The model under review builds one solid part; all positions refer to its coordinate system, in mm. Round coordinates to 2 decimals unless told otherwise and drop trailing zeros. Loops run counter-clockwise (first coordinate to the right, second up) from the corner with the lowest first, then second, coordinate; pieces in that order, holes last. Notation, with made-up numbers: (36, 14.25) -> (84, 14.25) arc R19 cw to (84, 24.25) -> close; hole circle Ø8 at (65, 22.5). An arc over 180 degrees is marked (long way). Use a Markdown table: item, result. Add a question column.
1) Wall thickness on probe 1 along Z at (x, y) = (-1, 1.25); probe 2 along Y at (x, z) = (7, 2.35); probe 3 along Y at (x, z) = (12, 0.95): over which ranges is each line inside the solid? List them lowest first.
2) Insertion check: pin 1 (2 mm diameter, centred on x = -9.5, y = -7.5, fed in from +Z); pin 2 (1 mm diameter, centred on y = 9.5, z = 1.5, fed in from +X); pin 3 (0.7 mm diameter, centred on x = -24, z = 1, fed in from -Y). Each pin has a flat end and moves straight along its axis. Give the tip position at first contact, or say it passes through.
3) Consider section B-B on x = -2. Give the boundary of the cut face in (y, z), plus the area to 3 significant figures.
4) Consider section A-A on x = -11. Give the boundary of the cut face in (y, z).
5) Mouldability with a two-part tool opening along X and no side actions: class faces 1 (the cylindrical face through (-21.37, -2.9, 0.8)), 2 (the flat face through (1, 0, 0)) as released by +X, released by -X, zero draft, split by the parting line, or undercut.
from build123d import *

# Parameters (mm, degrees)
SKETCH_W      = 7
SKETCH_H      = 7
PAD_DEPTH     = 2
FILLET_R      = 4
FILLET001_R   = 8
FILLET002_R   = 2
FILLET003_R   = 3
SKETCH001_W   = 33
SKETCH001_H   = 2
SKETCH001_W_2 = 4
PAD001_DEPTH  = 1
FILLET004_R   = 4
CHAMFER_SIZE  = 0.9
FILLET005_R   = 0.9
FILLET006_R   = 0.9
FILLET007_R   = 0.9
FILLET008_R   = 0.5
FILLET009_R   = 0.5
FILLET010_R   = 0.5


with BuildPart() as part:
    # Sketch → Pad (new body)
    with BuildSketch(Plane.XY):
        Polygon((-11.80015, 8), (32.19985, 8), (32.19985, -8), (-11.80015, -8), (-11.80015, -14), (-30.80015, -14), (-30.80015, 14), (-11.80015, 14), align=None)
        with Locations((-24.30015, 0)):
            Rectangle(SKETCH_W, SKETCH_H, mode=Mode.SUBTRACT)
    extrude(amount=PAD_DEPTH)

    # Fillet
    fillet_edges = [part.edges().sort_by_distance(p)[0] for p in [
        (-11.80015, -14, 1),
        (-11.80015, 14, 1),
    ]]
    fillet(fillet_edges, radius=FILLET_R)

    # Fillet001
    fillet001_edges = [part.edges().sort_by_distance(p)[0] for p in [
        (-30.80015, -14, 1),
        (-30.80015, 14, 1),
    ]]
    fillet(fillet001_edges, radius=FILLET001_R)

    # Fillet002
    fillet002_edges = [part.edges().sort_by_distance(p)[0] for p in [
        (-20.80015, -3.5, 1),
        (-20.80015, 3.5, 1),
        (-27.80015, 3.5, 1),
        (-27.80015, -3.5, 1),
    ]]
    fillet(fillet002_edges, radius=FILLET002_R)

    # Fillet003
    fillet003_edges = [part.edges().sort_by_distance(p)[0] for p in [
        (32.19985, -8, 1),
    ]]
    fillet(fillet003_edges, radius=FILLET003_R)

    # Sketch001 → Pad001 (new body)
    with BuildSketch(Plane.XY.offset(2)):
        with Locations((7.69985, 0)):
            Rectangle(SKETCH001_W, SKETCH001_H)
        with Locations((28.69985, 0)):
            Rectangle(SKETCH001_W_2, SKETCH001_H)
    extrude(amount=PAD001_DEPTH)

    # Fillet004
    fillet004_edges = [part.edges().sort_by_distance(p)[0] for p in [
        (32.19985, 8, 1),
    ]]
    fillet(fillet004_edges, radius=FILLET004_R)

    # Chamfer
    chamfer_edges = [part.edges().sort_by_distance(p)[0] for p in [
        (-8.80015, 0, 3),
        (24.19985, 0, 3),
        (26.69985, 0, 3),
        (30.69985, 0, 3),
    ]]
    chamfer(chamfer_edges, length=CHAMFER_SIZE)

    # Fillet005
    fillet005_edges = [part.edges().sort_by_distance(p)[0] for p in [
        (8.69985, -8, 2),
        (31.32117, -7.12132, 2),
        (32.19985, -0.5, 2),
        (31.028277, 6.828427, 2),
        (8.19985, 8, 2),
        (-11.80015, -9, 2),
        (-12.971723, -12.828427, 2),
        (-19.30015, -14, 2),
        (-28.457005, -11.656854, 2),
        (-30.80015, 0, 2),
        (-28.457005, 11.656854, 2),
        (-19.30015, 14, 2),
        (-12.971723, 12.828427, 2),
        (-11.80015, 9, 2),
    ]]
    fillet(fillet005_edges, radius=FILLET005_R)

    # Fillet006
    fillet006_edges = [part.edges().sort_by_distance(p)[0] for p in [
        (-21.385937, 2.914214, 2),
        (-20.80015, 0, 2),
        (-21.385937, -2.914214, 2),
        (-24.30015, -3.5, 2),
        (-27.214364, -2.914214, 2),
        (-27.80015, 0, 2),
        (-27.214364, 2.914214, 2),
        (-24.30015, 3.5, 2),
    ]]
    fillet(fillet006_edges, radius=FILLET006_R)

    # Fillet007
    fillet007_edges = [part.edges().sort_by_distance(p)[0] for p in [
        (8.69985, -8, 0),
        (31.32117, -7.12132, 0),
        (32.19985, -0.5, 0),
        (31.028277, 6.828427, 0),
        (8.19985, 8, 0),
        (-11.80015, 9, 0),
        (-12.971723, 12.828427, 0),
        (-19.30015, 14, 0),
        (-28.457005, 11.656854, 0),
        (-30.80015, 0, 0),
        (-28.457005, -11.656854, 0),
        (-19.30015, -14, 0),
        (-12.971723, -12.828427, 0),
        (-11.80015, -9, 0),
    ]]
    fillet(fillet007_edges, radius=FILLET007_R)

    # Fillet008
    fillet008_edges = [part.edges().sort_by_distance(p)[0] for p in [
        (-27.80015, 0, 0),
        (-27.214364, -2.914214, 0),
        (-24.30015, -3.5, 0),
        (-21.385937, -2.914214, 0),
        (-20.80015, 0, 0),
        (-21.385937, 2.914214, 0),
        (-24.30015, 3.5, 0),
        (-27.214364, 2.914214, 0),
    ]]
    fillet(fillet008_edges, radius=FILLET008_R)

    # Fillet009
    fillet009_edges = [part.edges().sort_by_distance(p)[0] for p in [
        (28.69985, -1, 3),
        (27.14985, -1, 2.55),
        (27.14985, 1, 2.55),
        (28.69985, 1, 3),
        (30.24985, 1, 2.55),
        (30.24985, -1, 2.55),
    ]]
    fillet(fillet009_edges, radius=FILLET009_R)

    # Fillet010
    fillet010_edges = [part.edges().sort_by_distance(p)[0] for p in [
        (7.69985, -1, 3),
        (7.69985, 1, 3),
        (23.74985, 1, 2.55),
        (23.74985, -1, 2.55),
        (-8.35015, -1, 2.55),
        (-8.35015, 1, 2.55),
    ]]
    fillet(fillet010_edges, radius=FILLET010_R)


solid = part.part
Result set:
| question | item | result |
|---|---|---|
| 1 | probe 1 | 0 to 2 |
| 1 | probe 2 | -1 to 1 |
| 1 | probe 3 | -8 to 8 |
| 2 | pin 1 | z = 2 |
| 2 | pin 2 | x = -11.8 |
| 2 | pin 3 | y = -13.95 |
| 3 | outline | (-8, 0.9) arc R0.9 ccw to (-7.1, 0) -> (7.1, 0) arc R0.9 ccw to (8, 0.9) -> (8, 1.1) arc R0.9 ccw to (7.1, 2) -> (1, 2) -> (1, 2.5) arc R0.5 ccw to (0.5, 3) -> (-0.5, 3) arc R0.5 ccw to (-1, 2.5) -> (-1, 2) -> (-7.1, 2) arc R0.9 ccw to (-8, 1.1) -> close |
| 3 | area | 33.2 mm2 |
| 4 | outline | (-8, 0.9) arc R0.9 ccw to (-7.1, 0) -> (7.1, 0) arc R0.9 ccw to (8, 0.9) -> (8, 1.1) arc R0.9 ccw to (7.1, 2) -> (-7.1, 2) arc R0.9 ccw to (-8, 1.1) -> close |
| 5 | face 1 | undercut |
| 5 | face 2 | zero draft |
